from build123d import *

# Parameters (mm, degrees)
EXTRUDE_1_DEPTH          = 3.5
EXTRUDE_2_DEPTH          = 2.6
PATTERN_CIRCULAR_1_COUNT = 2
PATTERN_CIRCULAR_1_ANGLE = 60
PATTERN_CIRCULAR_2_COUNT = 2
PATTERN_CIRCULAR_2_ANGLE = 60
EXTRUDE_3_DEPTH          = 3.5


with BuildPart() as part:
    # 草图1 → 凸台-拉伸1 (new body)
    with BuildSketch(Plane(origin=(0, 0, 0), x_dir=(1, 0, 0), z_dir=(0, 1, 0))):
        with BuildLine():
            Line((-2.6, 22.563332941), (2.6, 22.563332941))
            Line((2.6, 22.563332941), (2.6, 14.163332941))
            ThreePointArc((2.6, 14.163332941), (7.2, 12.470765814), (10.965806129, 9.33333252))
            Line((10.965806129, 9.33333252), (18.240419521, 13.53333252))
            Line((18.240419521, 13.53333252), (20.840419521, 9.030000421))
            Line((20.840419521, 9.030000421), (13.565806129, 4.830000421))
            ThreePointArc((13.565806129, 4.830000421), (0, -14.4), (-13.565806129, 4.830000421))
            Line((-13.565806129, 4.830000421), (-20.840419521, 9.030000421))
            Line((-20.840419521, 9.030000421), (-18.240419521, 13.53333252))
            Line((-18.240419521, 13.53333252), (-10.965806129, 9.33333252))
            ThreePointArc((-10.965806129, 9.33333252), (-7.2, 12.470765814), (-2.6, 14.163332941))
            Line((-2.6, 14.163332941), (-2.6, 22.563332941))
        make_face()
        with BuildLine():
            Line((4.596194078, 6.717514421), (2.243882157, 4.3652025))
            ThreePointArc((2.243882157, 4.3652025), (1.77992131, 4.102319563), (1.246817757, 4.115269794))
            ThreePointArc((1.246817757, 4.115269794), (0, 4.3), (-1.246817757, 4.115269794))
            ThreePointArc((-1.246817757, 4.115269794), (-1.77992131, 4.102319563), (-2.243882157, 4.3652025))
            Line((-2.243882157, 4.3652025), (-4.596194078, 6.717514421))
            ThreePointArc((-4.596194078, 6.717514421), (-6.717514421, 6.717514421), (-6.717514421, 4.596194078))
            Line((-6.717514421, 4.596194078), (-4.3652025, 2.243882157))
            ThreePointArc((-4.3652025, 2.243882157), (-4.102319563, 1.77992131), (-4.115269794, 1.246817757))
            ThreePointArc((-4.115269794, 1.246817757), (-4.3, 0), (-4.115269794, -1.246817757))
            ThreePointArc((-4.115269794, -1.246817757), (-4.102319563, -1.77992131), (-4.3652025, -2.243882157))
            Line((-4.3652025, -2.243882157), (-6.717514421, -4.596194078))
            ThreePointArc((-6.717514421, -4.596194078), (-6.717514421, -6.717514421), (-4.596194078, -6.717514421))
            Line((-4.596194078, -6.717514421), (-2.243882157, -4.3652025))
            ThreePointArc((-2.243882157, -4.3652025), (-1.77992131, -4.102319563), (-1.246817757, -4.115269794))
            ThreePointArc((-1.246817757, -4.115269794), (0, -4.3), (1.246817757, -4.115269794))
            ThreePointArc((1.246817757, -4.115269794), (1.77992131, -4.102319563), (2.243882157, -4.3652025))
            Line((2.243882157, -4.3652025), (4.596194078, -6.717514421))
            ThreePointArc((4.596194078, -6.717514421), (6.717514421, -6.717514421), (6.717514421, -4.596194078))
            Line((6.717514421, -4.596194078), (4.3652025, -2.243882157))
            ThreePointArc((4.3652025, -2.243882157), (4.102319563, -1.77992131), (4.115269794, -1.246817757))
            ThreePointArc((4.115269794, -1.246817757), (4.3, 0), (4.115269794, 1.246817757))
            ThreePointArc((4.115269794, 1.246817757), (4.102319563, 1.77992131), (4.3652025, 2.243882157))
            Line((4.3652025, 2.243882157), (6.717514421, 4.596194078))
            ThreePointArc((6.717514421, 4.596194078), (6.717514421, 6.717514421), (4.596194078, 6.717514421))
        make_face(mode=Mode.SUBTRACT)
    extrude(amount=EXTRUDE_1_DEPTH)

    # 草图2 → 凸台-拉伸2 (add, symmetric)
    with BuildSketch(Plane(origin=(0, 0, 0), x_dir=(0, 0, -1), z_dir=(1, 0, 0))):
        Polygon((22.563332941, 3.5), (33.063332941, 10), (74.4, 21.673878936), (74.4, 28.46), (78.6, 28.46), (78.6, 19.36), (33.063332941, 6.5), (22.563332941, 0), align=None)
    extrude_2 = extrude(amount=EXTRUDE_2_DEPTH, both=True)

    # 阵列(圆周)1: 凸台-拉伸2 ×2 about axis
    pattern_circular_1_axis = Axis((0, 3.5, 0), (0, 1, 0))
    for i in range(1, PATTERN_CIRCULAR_1_COUNT):
        add(extrude_2.rotate(pattern_circular_1_axis, i * PATTERN_CIRCULAR_1_ANGLE / (PATTERN_CIRCULAR_1_COUNT - 1)))

    # 阵列(圆周)2: 凸台-拉伸2 ×2 about axis
    pattern_circular_2_axis = Axis((0, 3.5, 0), (0, -1, 0))
    for i in range(1, PATTERN_CIRCULAR_2_COUNT):
        add(extrude_2.rotate(pattern_circular_2_axis, i * PATTERN_CIRCULAR_2_ANGLE / (PATTERN_CIRCULAR_2_COUNT - 1)))

    # 草图3 → 凸台-拉伸3 (add)
    with BuildSketch(Plane(origin=(0, 28.46, 0), x_dir=(1, 0, 0), z_dir=(0, 1, 0))):
        with BuildLine():
            Line((-69.369596737, 37.04833395), (-65.732290042, 34.94833395))
            ThreePointArc((-65.732290042, 34.94833395), (0, 74.445416246), (65.732290042, 34.94833395))
            Line((65.732290042, 34.94833395), (69.369596737, 37.04833395))
            ThreePointArc((69.369596737, 37.04833395), (0, 78.642990787), (-69.369596737, 37.04833395))
        make_face()
    extrude(amount=EXTRUDE_3_DEPTH)


solid = part.part
Work out the finished part from the listing and answer in its coordinate system (mm). A direction names the side the tool comes from. Coordinates: 2 decimals unless noted, no trailing zeros. Write each loop counter-clockwise with the first axis right and the second up, starting at its lowest first coordinate (ties: lowest second). Pieces come first, ordered by that corner, then holes. Notation, with made-up numbers: (50.25, 41) - (54.25, 41) arc R24 ccw to (54.25, 63) - close; hole circle Ø8 at (-36.75, -22.75). An arc over 180 degrees is marked (long way). One line per question, with ' | ' between items.
1) For faces 5 (the face through (24.042, 6.704, -13.838)), 6 (the face through (48.65, 13.02, -28.04)), determine the directions among +Z, -Z, +X, -X, +Y, -Y from which every point of the face is accessible in a straight line to the end or side of a thin tool.
Checks:
face 5: +Z, +Y | face 6: -Z, +X, -Y
2) The mould has two halves that part along X. Classify faces 1 (the face through (-6.694, 1.726, -6.741)), 2 (the face through (46.301, 15.755, -26.69)), 3 (the face through (0.036, 15.755, -53.442)), 4 (the face through (0.386, 1.726, 14.395)): +X half, -X half, draft (parallel to the pull), parting line (faces both ways), or undercut.
Checks:
face 1: undercut | face 2: undercut | face 3: draft | face 4: parting line
3) Find section A-A, the plane z = -67.5. Determine the outline of the cut face in (x, y), and give its area (3 significant figures).
Checks:
outline: (-40.35, 28.46) - (-31.4, 28.46) - (-31.4, 31.96) - (-40.35, 31.96) - close; (-2.6, 16.23) - (2.6, 16.23) - (2.6, 19.73) - (-2.6, 19.73) - close; (31.4, 28.46) - (40.35, 28.46) - (40.35, 31.96) - (31.4, 31.96) - close | area: 80.9 mm2
4) Find section B-B, the plane x = -35. Determine the outline of the cut face in (y, z), and give its area (3 significant figures).
Checks:
outline: (8.15, -17.21) - (9, -23.21) - (12.5, -23.21) - (11.65, -17.21) - close; (28.46, -70.43) - (31.96, -70.43) - (31.96, -65.7) - (28.46, -65.7) - close | area: 37.5 mm2
5) Consider probe 1 along X at (y, z) = (18.5, -70.5); probe 2 along X at (y, z) = (29.5, -46); probe 3 along Z at (x, y) = (58, 17.5). Determine where each line is inside the solid, lowest interval first. Write a range as [from, to].
Checks:
probe 1: [-2.6, 2.6] | probe 2: [-63.79, -58.53], [58.53, 63.79] | probe 3: [-36.49, -30.48]
6) Find section C-C, the plane y = 16.5. Determine the outline of the cut face in (x, z).
Checks:
outline: (-60.6, -31.98) - (-58, -36.49) - (-47.27, -30.29) - (-49.87, -25.79) - close; (-2.6, -68.47) - (2.6, -68.47) - (2.6, -56.08) - (-2.6, -56.08) - close; (47.27, -30.29) - (58, -36.49) - (60.6, -31.98) - (49.87, -25.79) - close
7) Flat-ended cylindrical pins translate along their axes: P1, Ø12, axis at y = 24, z = -37, coming from the +X side; P2, Ø14, axis at y = 12, z = -52.5, coming from the +X side; P3, Ø3, axis at x = 67.5, z = -38, coming from the -Y side; P4, Ø8.5, axis at y = 12.5, z = -51.5, coming from the -X side. Find the tip coordinate at first contact, or state that the pin passes through.
Checks:
P1: x = 69.37 | P2: x = 2.6 | P3: y = 18.61 | P4: x = -2.6
